```python
from build123d import *

# Parameters (mm, degrees)
FILLET1_R           = 10
LPATTERN2_COUNT     = 2
LPATTERN2_PITCH     = 300
LPATTERN3_COUNT     = 2
LPATTERN3_PITCH     = 300
SKETCH2_W           = 500
SKETCH2_H           = 500
BOSS_EXTRUDE1_DEPTH = 15
BOSS_EXTRUDE1_TAPER = 30
FILLET2_R           = 80


with BuildPart() as part:
    # Sketch1 → Revolve1 (revolve)
    with BuildSketch(Plane.XY, mode=Mode.PRIVATE) as revolve1_sk:
        with BuildLine():
            Line((0, 200), (0, 0))
            Line((0, 0), (25, 0))
            ThreePointArc((25, 0), (35.658376663, 11.181839274), (35.288232701, 26.625204065))
            Line((35.288232701, 26.625204065), (20, 26.625204065))
            ThreePointArc((20, 26.625204065), (23.557403108, 113.312602033), (20, 200))
            Line((20, 200), (0, 200))
        make_face()
    revolve(revolve1_sk.sketch.rotate(Axis((0, 200, 0), (0, -1, 0)), 180), axis=Axis((0, 200, 0), (0, -1, 0)))

    # Fillet1
    fillet1_edges = [part.edges().sort_by_distance(p)[0] for p in [
        (35.288232701, 26.625204065, 0),
    ]]
    fillet(fillet1_edges, radius=FILLET1_R)


with BuildPart() as lpattern2_1:
    # LPattern2: pattern copy
    add(part.part.moved(Location(Vector(0, 0, -1) * (1 * LPATTERN2_PITCH))))


with BuildPart() as lpattern3_1:
    # LPattern3: pattern copy
    add(lpattern2_1.part.moved(Location(Vector(-1, 0, 0) * (1 * LPATTERN3_PITCH))))


with BuildPart() as lpattern3_2:
    # LPattern3: pattern copy
    add(part.part.moved(Location(Vector(-1, 0, 0) * (1 * LPATTERN3_PITCH))))


with BuildPart() as part_1:
    add(part.part)

    add(lpattern2_1.part)  # Boss-Extrude1 merges LPattern2_1

    add(lpattern3_1.part)  # Boss-Extrude1 merges LPattern3_1

    add(lpattern3_2.part)  # Boss-Extrude1 merges LPattern3_2
    # Sketch2 → Boss-Extrude1 (add)
    with BuildSketch(Plane(origin=(0, 200, 0), x_dir=(1, 0, 0), z_dir=(0, 1, 0))):
        with Locations((-150, 150)):
            Rectangle(SKETCH2_W, SKETCH2_H)
    extrude(amount=BOSS_EXTRUDE1_DEPTH, taper=BOSS_EXTRUDE1_TAPER)

    # Fillet2
    # the kernel refuses this fillet: 80 mm, written as the material it takes off along each edge
    with BuildSketch(Plane(origin=(-469.282032303, 80, -469.282032303), x_dir=(-0.22360679774997919, -0.3872983346207402, 0.8944271909999165), z_dir=(0.44721359549995965, 0.774596669241483, 0.4472135954999567)), Plane(origin=(169.282032303, 80, -469.282032303), x_dir=(-0.8944271909999159, -0.38729833462074126, -0.22360679774997977), z_dir=(-0.4472135954999579, 0.7745966692414825, 0.4472135954999594))) as fillet2_piece_1:
        with BuildLine():
            CenterArc((FILLET2_R * 0.774596669241, FILLET2_R), FILLET2_R, 194.477512186, 75.522487814)
            Line((-FILLET2_R * 0.19364916731, FILLET2_R * 0.75), (0, 0))
            Line((0, 0), (FILLET2_R * 0.774596669241, 0))
        make_face()
    extrude(amount=329.203584428, mode=Mode.SUBTRACT)
    with BuildSketch(Plane(origin=(-469.282032303, 80, 169.282032303), x_dir=(-0.22360679774998043, -0.38729833462074226, -0.8944271909999153), z_dir=(0.4472135954999591, 0.774596669241482, -0.4472135954999591)), Plane(origin=(169.282032303, 80, 169.282032303), x_dir=(-0.8944271909999149, -0.387298334620743, 0.22360679774998055), z_dir=(-0.4472135954999599, 0.774596669241482, -0.4472135954999584))) as fillet2_piece_2:
        with BuildLine():
            CenterArc((FILLET2_R * 0.774596669241, -FILLET2_R), FILLET2_R, 90, 75.522487814)
            Line((-FILLET2_R * 0.19364916731, -FILLET2_R * 0.75), (0, 0))
            Line((0, 0), (FILLET2_R * 0.774596669241, 0))
        make_face()
    extrude(amount=329.203584428, mode=Mode.SUBTRACT)


solid = part_1.part
```
The listing builds one solid part. Answer for the finished solid, in the listing's coordinates (mm). A direction names the side the tool comes from. Give positions to 0.01 mm unless a question says otherwise; leave off trailing zeros. Answer as CSV lines item,"result". Start each with the question number.
Item 1: The mould has two halves that part along Z. Classify faces 1 (the face through (-290, 26.625, 18)), 2 (the face through (-374.358, 211.803, 73.314)), 3 (the face through (0, 0, -300)): +Z half, -Z half, draft (parallel to the pull), parting line (faces both ways), or undercut.
Item 2: Each of these flat-tipped pins is pushed along its axis until it touches: pin 1 (5 mm diameter, centred on x = -12.5, y = 171.5, fed in from -Z); pin 2 (5 mm diameter, centred on y = 50, z = -290.5, fed in from +X); pin 3 (6 mm diameter, centred on x = -166.5, z = 38, fed in from -Y). Where does it stop, or does it pass through?
Item 3: Find the intervals of material crossed by line 1 (Y direction, x = -303, z = -172.5); line 2 (X direction, y = 76, z = -288); line 3 (Y direction, x = 25, z = 5.5), in increasing order. Write a range as from..to.
Item 4: For faces 4 (the face through (10, 26.625, 18)), 5 (the face through (0, 0, 0)), determine the directions among +Z, -Z, +X, -X, +Y, -Y from which every point of the face is accessible in a straight line to the end or side of a thin tool.
Found:
1,face 1,"undercut"
1,face 2,"+Z half"
1,face 3,"draft"
2,pin 1,"stops at z = -319.56"
2,pin 2,"stops at x = 20.51"
2,pin 3,"stops at y = 200"
3,line 1,"y = 200..215"
3,line 2,"x = -319.5..-280.5, -19.5..19.5"
3,line 3,"y = 0.28..26.63, 200..215"
4,face 4,"none"
4,face 5,"+Z, -Z, +X, -X, -Y"
